For this review, use the dimensioned drawing (mm, ordinates from the lowest corner) and the shaded views. A direction names the side the tool comes from. Give positions to 0.01 mm unless a question says otherwise; leave off trailing zeros. Order: outer loops, then holes, each group sorted by start corner. A loop starts at its lowest first (then second) coordinate and runs counter-clockwise, first axis right, second up.
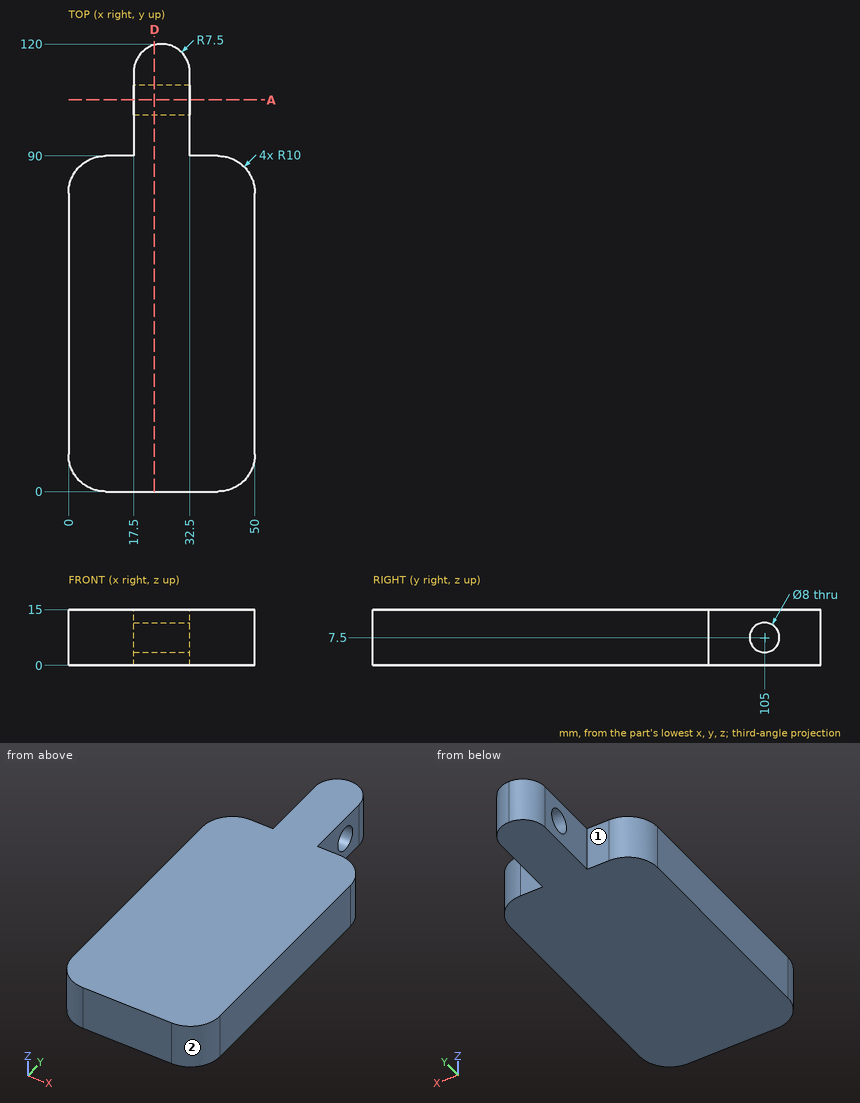
1. Take a section at A-A (y = 105). State the section outline as (x, z) points.
Recorded:
outline: (17.5, 0) - (32.5, 0) - (32.5, 3.5) - (17.5, 3.5) - close; (17.5, 11.5) - (32.5, 11.5) - (32.5, 15) - (17.5, 15) - close
2. Take a section at D-D (x = 23). State the section outline as (y, z) points, then the cut area to 3 significant figures.
Recorded:
outline: (0, 0) - (119.73, 0) - (119.73, 15) - (0, 15) - close; hole circle Ø8 at (105, 7.5)
area: 1,750 mm2
3. For line 1 along Z through (x, y) = (21, 105); line 2 along Y through (x, z) = (34.5, 10.5); line 3 along Y through (x, z) = (31, 5.5), list the stretches that pass through material, from the lowest coordinate up.
Recorded:
line 1: z = 0 to 3.5, 11.5 to 15
line 2: y = 0 to 90
line 3: y = 0 to 101.54, 108.46 to 117
4. Machinability: for the marked faces 1 and 2, which of the approach directions +Z, -Z, +X, -X, +Y, -Y give a long, thin tool a straight path to every point of the face, cutting with its end or side? Answer none if there is none.
Recorded:
face 1: +Z, -Z, -X, +Y
face 2: +Z, -Z, +X, -Y
5. For pin 1 (5 mm diameter, centred on y = 105, z = 7.5, fed in from +X); pin 2 (1.5 mm diameter, centred on y = 86.5, z = 13.5, fed in from +X); pin 3 (6 mm diameter, centred on x = 6.5, z = 10, fed in from -Y); pin 4 (6 mm diameter, centred on x = 37, z = 7, fed in from +Y), all flat-tipped, find the tip position at first contact; note any pin that passes through.
Recorded:
pin 1: passes through
pin 2: stops at x = 48.18
pin 3: stops at y = 0.01
pin 4: stops at y = 90
